Here's how the part is built. I have some questions about the finished solid (model axes, mm). A direction names the side the tool comes from. Coordinates: 2 decimals unless noted, no trailing zeros. Write each loop counter-clockwise with the first axis right and the second up, starting at its lowest first coordinate (ties: lowest second). Pieces come first, ordered by that corner, then holes. Notation, with made-up numbers: (23, 86.25) -> (76, 86.25) arc R14 cw to (76, 91.25) -> close; hole circle Ø4 at (43, -25.75). An arc over 180 degrees is marked (long way). Put each result on its own line as item: value. Start each with the question number.
Item 1: I want a section at C-C, the plane y = 4.5. State how many separate pieces and enclosed holes the cut face has, then the cut area to 3 significant figures.
Item 2: I want a section at B-B, the plane x = 16. List the corners of the cut face in (y, z) for me.
Item 3: I want a section at A-A, the plane x = -5. List the corners of the cut face in (y, z) for me, then the cut area to 3 significant figures.
Item 4: If we mould it in two halves opening along X, with no side actions, what happens to faces 1 (the face through (9, 0, 42)), 2 (the face through (-8, 3.5, 34)), 3 (the face through (23.7, 3.61, 51.42))? For each: released by +X, released by -X, zero draft, split by the parting line, or undercut.
Item 5: For pin 1 (2 mm diameter, centred on x = -9, z = 34, fed in from +Y); pin 2 (5.5 mm diameter, centred on x = -9.76, z = 4.46, fed in from -Y); pin 3 (2.5 mm diameter, centred on x = -5.76, z = -11.54, fed in from +Y), each with a flat end and sliding along its axis, tell me the tip position at first contact or that it passes through.
Item 6: I want a section at D-D, the plane x = -10. List the corners of the cut face in (y, z) for me.
Item 7: I need wall thicknesses on line 1 (Z direction, x = 2.5, y = 0.25); line 2 (X direction, y = 4, z = 24); line 3 (Z direction, x = 5, y = 4). Which ranges of each line are inside material? Lowest first, please. Write a range as [from, to].
Item 8: On a 3-axis mill with a long thin cutter (end or side, diameter ignored), from which of +Z, -Z, +X, -X, +Y, -Y can I reach the whole of each face in a straight line? I mean faces 4 (the face through (9, 0, -5)), 5 (the face through (-10.179, 5.274, 29.242)), 6 (the face through (-3.82, 3.45, 48.51)). Say none if no direction works.
from build123d import *

# Parameters (mm, degrees)
SKETCH1_W             = 50
SKETCH1_H             = 76.6
SKETCH1_R             = 6.5
SKETCH1_R_2           = 1.75
SKETCH1_R_3           = 1.5
BOSS_EXTRUDE1_DEPTH   = 7
M5_TAPPED_HOLE1_D     = 4.2
M5_TAPPED_HOLE1_DEPTH = 10
M5_TAPPED_HOLE1_TIP   = 1.2618073
SKETCH4_R             = 3.25
CUT_EXTRUDE1_DEPTH    = 3.5
M3_TAPPED_HOLE1_D     = 2.5
M3_TAPPED_HOLE1_DEPTH = 20
M3_TAPPED_HOLE1_TIP   = 0.751075774
SKETCH10_W            = 50
SKETCH10_H            = 18
CUT_EXTRUDE3_DEPTH    = 1
SKETCH11_W            = 50
SKETCH11_H            = 16
BOSS_EXTRUDE2_DEPTH   = 3.5
M3_TAPPED_HOLE2_D     = 2.5
M3_TAPPED_HOLE2_DEPTH = 20
M3_TAPPED_HOLE2_TIP   = 0.751075774


with BuildPart() as part:
    # Sketch1 → Boss-Extrude1 (new body)
    with BuildSketch(Plane(origin=(0, 0, 0), x_dir=(1, 0, 0), z_dir=(0, 1, 0))):
        with Locations((9.743944876, -18.464670659)):
            Rectangle(SKETCH1_W, SKETCH1_H)
        with Locations((24.714004756, -0.164670659)):
            Circle(SKETCH1_R, mode=Mode.SUBTRACT)
        with Locations((24.714004756, -36.164670659)):
            Circle(SKETCH1_R, mode=Mode.SUBTRACT)
        with Locations((-9.756055124, -4.464670659)):
            Circle(SKETCH1_R_2, mode=Mode.SUBTRACT)
        with Locations((-9.756055124, -32.464670659)):
            Circle(SKETCH1_R_2, mode=Mode.SUBTRACT)
        with Locations((-5.756055124, -48.464670659)):
            Circle(SKETCH1_R_3, mode=Mode.SUBTRACT)
        with Locations((-5.756055124, 11.535329341)):
            Circle(SKETCH1_R_3, mode=Mode.SUBTRACT)
        with BuildLine():
            Line((-1.568862275, 13.785329341), (8.431137725, 13.785329341))
            ThreePointArc((8.431137725, 13.785329341), (10.681137725, 11.535329341), (8.431137725, 9.285329341))
            Line((8.431137725, 9.285329341), (-1.568862275, 9.285329341))
            ThreePointArc((-1.568862275, 9.285329341), (-3.818862275, 11.535329341), (-1.568862275, 13.785329341))
        make_face(mode=Mode.SUBTRACT)
        with BuildLine():
            Line((-1.568862275, -46.214670659), (8.431137725, -46.214670659))
            ThreePointArc((8.431137725, -46.214670659), (10.681137725, -48.464670659), (8.431137725, -50.714670659))
            Line((8.431137725, -50.714670659), (-1.568862275, -50.714670659))
            ThreePointArc((-1.568862275, -50.714670659), (-3.818862275, -48.464670659), (-1.568862275, -46.214670659))
        make_face(mode=Mode.SUBTRACT)
    extrude(amount=BOSS_EXTRUDE1_DEPTH)

    # M5 Tapped Hole1
    with Locations(Plane(origin=(34.743944876, 0, 0), x_dir=(0, 0, -1), z_dir=(1, 0, 0))):
        with Locations((14.835829661, 3.5), (-51.764670659, 3.5)):
            Hole(M5_TAPPED_HOLE1_D / 2, depth=M5_TAPPED_HOLE1_DEPTH)
            with Locations((0, 0, -(M5_TAPPED_HOLE1_DEPTH + M5_TAPPED_HOLE1_TIP / 2))):  # 118° drill point
                Cone(0, M5_TAPPED_HOLE1_D / 2, M5_TAPPED_HOLE1_TIP, mode=Mode.SUBTRACT)

    # Sketch4 → Cut-Extrude1 (cut)
    with BuildSketch(Plane(origin=(0, 7, 0), x_dir=(1, 0, 0), z_dir=(0, 1, 0))):
        with Locations((-9.756055124, -4.464670659)):
            Circle(SKETCH4_R)
        with Locations((-9.756055124, -32.464670659)):
            Circle(SKETCH4_R)
    extrude(amount=-CUT_EXTRUDE1_DEPTH, mode=Mode.SUBTRACT)

    # M3 Tapped Hole1
    with Locations(Plane(origin=(0, 7, 0), x_dir=(1, 0, 0), z_dir=(0, 1, 0))):
        with Locations((20.243944876, -12.464670659), (28.243944876, -12.464670659), (28.243944876, -24.464670659), (20.243944876, -24.464670659)):
            Hole(M3_TAPPED_HOLE1_D / 2, depth=M3_TAPPED_HOLE1_DEPTH)
            with Locations((0, 0, -(M3_TAPPED_HOLE1_DEPTH + M3_TAPPED_HOLE1_TIP / 2))):  # 118° drill point
                Cone(0, M3_TAPPED_HOLE1_D / 2, M3_TAPPED_HOLE1_TIP, mode=Mode.SUBTRACT)

    # Sketch10 → Cut-Extrude3 (cut)
    with BuildSketch(Plane.XZ):
        with Locations((9.743944876, 18.464670659)):
            Rectangle(SKETCH10_W, SKETCH10_H)
    extrude(amount=-CUT_EXTRUDE3_DEPTH, mode=Mode.SUBTRACT)

    # Sketch11 → Boss-Extrude2 (add)
    with BuildSketch(Plane.XZ.offset(-1)):
        with Locations((9.743944876, 18.464670659)):
            Rectangle(SKETCH11_W, SKETCH11_H)
    extrude(amount=BOSS_EXTRUDE2_DEPTH)

    # M3 Tapped Hole2
    with Locations(Plane(origin=(0, -2.5, 0), x_dir=(-1, 0, 0), z_dir=(0, -1, 0))):
        with Locations((-20.243944876, -12.464670659), (-28.243944876, -12.464670659), (-20.243944876, -24.464670659), (-28.243944876, -24.464670659), (-47.068271945, 0)):
            Hole(M3_TAPPED_HOLE2_D / 2, depth=M3_TAPPED_HOLE2_DEPTH)
            with Locations((0, 0, -(M3_TAPPED_HOLE2_DEPTH + M3_TAPPED_HOLE2_TIP / 2))):  # 118° drill point
                Cone(0, M3_TAPPED_HOLE2_D / 2, M3_TAPPED_HOLE2_TIP, mode=Mode.SUBTRACT)


solid = part.part
Calculated:
1. separate pieces: 1
1. enclosed holes: 12
1. area: 3,270 mm2
2. outline: (-2.5, 10.46) -> (1, 10.46) -> (1, 9.46) -> (0, 9.46) -> (0, -19.84) -> (7, -19.84) -> (7, 56.76) -> (0, 56.76) -> (0, 27.46) -> (1, 27.46) -> (1, 26.46) -> (-2.5, 26.46) -> close
3. outline: (-2.5, 10.46) -> (1, 10.46) -> (1, 9.46) -> (0, 9.46) -> (0, -10.24) -> (7, -10.24) -> (7, 47.17) -> (0, 47.17) -> (0, 27.46) -> (1, 27.46) -> (1, 26.46) -> (-2.5, 26.46) -> close; (0, -19.84) -> (7, -19.84) -> (7, -12.83) -> (0, -12.83) -> close; (0, 49.76) -> (7, 49.76) -> (7, 56.76) -> (0, 56.76) -> close
3. area: 538 mm2
4. face 1: zero draft
4. face 2: undercut
4. face 3: released by +X
5. pin 1: stops at y = 3.5
5. pin 2: stops at y = 0
5. pin 3: passes through
6. outline: (-2.5, 10.46) -> (1, 10.46) -> (1, 9.46) -> (0, 9.46) -> (0, 6.2) -> (3.5, 6.2) -> (3.5, 7.71) -> (7, 7.71) -> (7, 29.22) -> (3.5, 29.22) -> (3.5, 30.73) -> (0, 30.73) -> (0, 27.46) -> (1, 27.46) -> (1, 26.46) -> (-2.5, 26.46) -> close; (0, -19.84) -> (7, -19.84) -> (7, 1.22) -> (3.5, 1.22) -> (3.5, 2.73) -> (0, 2.73) -> close; (0, 34.2) -> (3.5, 34.2) -> (3.5, 35.71) -> (7, 35.71) -> (7, 56.76) -> (0, 56.76) -> close
7. line 1: z = [-19.84, -13.79], [-9.29, 9.46], [10.46, 26.46], [27.46, 46.21], [50.71, 56.76]
7. line 2: x = [-15.26, 19.08], [21.4, 27.08], [29.4, 34.74]
7. line 3: z = [-19.84, -13.79], [-9.29, 46.21], [50.71, 56.76]
8. face 4: -Z, +X, -X, -Y
8. face 5: +Y
8. face 6: +Y, -Y
